Design review of the part built by this model. Coordinates are the model's own, in mm. Face numbers are marked on the shaded views. A direction names the side the tool comes from. Coordinates: 2 decimals unless noted, no trailing zeros.
Q1. The part is to be moulded in two halves that separate along X. For the marked faces 1, 2 and 3, say which applies: released by +X, released by -X, zero draft, split by the parting line, or undercut.
Q2. For pin 1 Ø1 at (x, z) = (12, -10.5) entering from +Y; pin 2 Ø11.5 at (x, y) = (2, 37) entering from -Z; pin 3 Ø0.6 at (x, z) = (1.5, 24.5) entering from +Y; pin 4 Ø3 at (y, z) = (5, 0) entering from +X, all flat-tipped, find the tip position at first contact; note any pin that passes through.
Q3. For the marked faces 4, 5 and 6, list the 3-axis set-ups (+Z, -Z, +X, -X, +Y, -Y) from which the entire face can be reached by the end or side of a thin tool; tool diameter is ignored.
Q4. For L1, parallel to Z at x = 22.45, y = 5 (3 decimals); L2, parallel to X at y = 8, z = 0; L3, parallel to X at y = 26, z = -15, list the stretches that pass through material, from the lowest coordinate up.
from build123d import *

# Parameters (mm, degrees)
SKETCH1_R               = 25
SKETCH1_R_2             = 20.15
BOSS_EXTRUDE1_DEPTH     = 10
SKETCH2_R               = 25
BOSS_EXTRUDE2_DEPTH     = 5
BOSS_EXTRUDE3_DEPTH     = 50
CUT_EXTRUDE1_DEPTH      = 50
SKETCH5_W               = 44
SKETCH5_H               = 33.5
CUT_EXTRUDE2_DEPTH      = 2.33
SKETCH6_W               = 31.902194282
SKETCH6_H               = 10.372222151
BOSS_EXTRUDE5_DEPTH     = 45
BOSS_EXTRUDE6_DEPTH     = 45
BOSS_EXTRUDE7_DEPTH     = 20
SKETCH10_R              = 1.375
CUT_EXTRUDE3_DEPTH      = 77
SKETCH11_R              = 1.375
CUT_EXTRUDE4_DEPTH      = 77
SKETCH12_R              = 3
CUT_EXTRUDE5_DEPTH      = 7.38
CUT_EXTRUDE6_DEPTH      = 7.88
CUT_EXTRUDE6_DEPTH_BACK = 7.38
SKETCH13_R              = 3
CHAMFER1_SIZE           = 30
CHAMFER1_SIZE_2         = 5.289809421
CUT_EXTRUDE7_DEPTH      = 37
CUT_EXTRUDE7_DEPTH_BACK = 37
SKETCH16_R              = 1.625


with BuildPart() as part:
    # Sketch1 → Boss-Extrude1 (new body)
    with BuildSketch(Plane(origin=(0, 0, 0), x_dir=(1, 0, 0), z_dir=(0, 1, 0))):
        with Locations(Location((0, 0, 0), (0, 0, 270))):
            Circle(SKETCH1_R)
        with Locations(Location((0, 0, 0), (0, 0, 270))):
            Circle(SKETCH1_R_2, mode=Mode.SUBTRACT)
    extrude(amount=BOSS_EXTRUDE1_DEPTH)

    # Sketch2 → Boss-Extrude2 (add)
    with BuildSketch(Plane(origin=(0, 10, 0), x_dir=(1, 0, 0), z_dir=(0, 1, 0))):
        with Locations(Location((0, 0, 0), (0, 0, 270))):
            Circle(SKETCH2_R)
    extrude(amount=BOSS_EXTRUDE2_DEPTH)

    # Sketch3 → Boss-Extrude3 (add)
    with BuildSketch(Plane(origin=(0, 15, 0), x_dir=(1, 0, 0), z_dir=(0, 1, 0))):
        with BuildLine():
            ThreePointArc((4.974937186, -24.5), (12.844564237, -21.448010853), (19.25, -15.951097141))
            Line((19.25, -15.951097141), (19.25, 15.951097141))
            ThreePointArc((19.25, 15.951097141), (12.844564237, 21.448010853), (4.974937186, 24.5))
            Line((4.974937186, 24.5), (-4.974937186, 24.5))
            ThreePointArc((-4.974937186, 24.5), (-12.844564237, 21.448010853), (-19.25, 15.951097141))
            Line((-19.25, 15.951097141), (-19.25, -15.951097141))
            ThreePointArc((-19.25, -15.951097141), (-12.844564237, -21.448010853), (-4.974937186, -24.5))
            Line((-4.974937186, -24.5), (4.974937186, -24.5))
        make_face()
    extrude(amount=BOSS_EXTRUDE3_DEPTH)

    # Sketch4 → Cut-Extrude1 (cut)
    with BuildSketch(Plane.XY.offset(24.5)):
        Polygon((-4.974937186, 44.974937186), (4.974937186, 35.025062814), (4.974937186, 65), (-4.974937186, 65), align=None)
        Polygon((4.974937186, 35.025062814), (25, 15), (25, 65), (4.974937186, 65), align=None)
        Polygon((-19.25, 59.25), (-4.974937186, 44.974937186), (-4.974937186, 65), (-19.25, 65), align=None)
    extrude(amount=-CUT_EXTRUDE1_DEPTH, mode=Mode.SUBTRACT)

    # Sketch5 → Cut-Extrude2 (cut)
    # profile 1 of 2: a face of its own
    with BuildSketch(Plane(origin=(20, 20, 0), x_dir=(0, 0, -1), z_dir=(0.7071067811865485, 0.7071067811865467, 0))):
        with BuildLine():
            Line((21.978674947, 45.132882323), (-21.978674947, 45.132882323))
            add(Edge.make_bspline(
                [(-21.978674947, 45.132882323), (-22.0399199, 44.9730967), (-22.1, 44.81242904)],
                knots=[4.215256564, 4.215256564, 4.215256564, 4.225444941, 4.225444941, 4.225444941], degree=2, weights=[0.971948047, 0.972055152, 0.97218796]))
            Line((-22.1, 44.81242904), (-22.1, 11.756113455))
            add(Edge.make_bspline(
                [(-22.1, 11.756113455), (-22.039397631, 11.594049133), (-21.977610099, 11.432882323)],
                knots=[5.19933302, 5.19933302, 5.19933302, 5.20960995, 5.20960995, 5.20960995], degree=2, weights=[0.97218796, 0.972053998, 0.971946187]))
            Line((-21.977610099, 11.432882323), (21.977610099, 11.432882323))
            add(Edge.make_bspline(
                [(21.977610099, 11.432882323), (22.039397631, 11.594049133), (22.1, 11.756113455)],
                knots=[1.073575357, 1.073575357, 1.073575357, 1.083852287, 1.083852287, 1.083852287], degree=2, weights=[0.971946187, 0.972053998, 0.97218796]))
            Line((22.1, 11.756113455), (22.1, 44.81242904))
            add(Edge.make_bspline(
                [(22.1, 44.81242904), (22.0399199, 44.9730967), (21.978674947, 45.132882323)],
                knots=[2.057740366, 2.057740366, 2.057740366, 2.067928743, 2.067928743, 2.067928743], degree=2, weights=[0.97218796, 0.972055152, 0.971948047]))
        make_face()
        with Locations((0, 28.282882323)):
            Rectangle(SKETCH5_W, SKETCH5_H, mode=Mode.SUBTRACT)
    # profile 2 of 2: a face of its own
    with BuildSketch(Plane(origin=(20, 20, 0), x_dir=(0, 0, -1), z_dir=(0.7071067811865485, 0.7071067811865467, 0))):
        with Locations((0, 28.282882323)):
            Rectangle(SKETCH5_W, SKETCH5_H)
    extrude(amount=-CUT_EXTRUDE2_DEPTH, mode=Mode.SUBTRACT)

    # Sketch6 → Boss-Extrude5 (add)
    with BuildSketch(Plane(origin=(20, 20, 0), x_dir=(0, 0, -1), z_dir=(0.7071067811865487, 0.7071067811865465, 0))):
        with BuildLine():
            Line((-15.951097141, 1.060660172), (-15.951097141, 11.432882323))
            Line((-15.951097141, 11.432882323), (-21.977610099, 11.432882323))
            add(Edge.make_bspline(
                [(-21.977610099, 11.432882323), (-19.67346685, 5.422747233), (-15.951097141, 1.060660172)],
                knots=[5.209205396, 5.209205396, 5.209205396, 5.591230132, 5.591230132, 5.591230132], degree=2, weights=[1, 0.981812537, 1]))
        make_face()
        with Locations((0, 6.246771248)):
            Rectangle(SKETCH6_W, SKETCH6_H)
        with BuildLine():
            Line((21.977610099, 11.432882323), (15.951097141, 11.432882323))
            Line((15.951097141, 11.432882323), (15.951097141, 1.060660172))
            add(Edge.make_bspline(
                [(15.951097141, 1.060660172), (19.67346685, 5.422747233), (21.977610099, 11.432882323)],
                knots=[0.691955175, 0.691955175, 0.691955175, 1.073979912, 1.073979912, 1.073979912], degree=2, weights=[1, 0.981812537, 1]))
        make_face()
    extrude(amount=BOSS_EXTRUDE5_DEPTH)

    # Sketch7 → Boss-Extrude6 (add)
    with BuildSketch(Plane(origin=(20, 20, 0), x_dir=(0, 0, -1), z_dir=(0.7071067811865487, 0.7071067811865465, 0))):
        with BuildLine():
            Line((15.951097141, 55.507882323), (-15.951097141, 55.507882323))
            add(Edge.make_bspline(
                [(-15.951097141, 55.507882323), (-19.67435923, 51.144749519), (-21.978674947, 45.132882323)],
                knots=[3.833547829, 3.833547829, 3.833547829, 4.215661937, 4.215661937, 4.215661937], degree=2, weights=[1, 0.981804052, 1]))
            Line((-21.978674947, 45.132882323), (21.978674947, 45.132882323))
            add(Edge.make_bspline(
                [(21.978674947, 45.132882323), (19.67435923, 51.144749519), (15.951097141, 55.507882323)],
                knots=[2.06752337, 2.06752337, 2.06752337, 2.449637478, 2.449637478, 2.449637478], degree=2, weights=[1, 0.981804052, 1]))
        make_face()
    extrude(amount=BOSS_EXTRUDE6_DEPTH)

    # Sketch8 → Boss-Extrude7 (add)
    with BuildSketch(Plane(origin=(0, 15, 0), x_dir=(1, 0, 0), z_dir=(0, 1, 0))):
        with BuildLine():
            ThreePointArc((25, 0), (23.518609653, 8.477912479), (19.25, 15.951097141))
            Line((19.25, 15.951097141), (19.25, -15.951097141))
            ThreePointArc((19.25, -15.951097141), (23.518609653, -8.477912479), (25, 0))
        make_face()
    extrude(amount=BOSS_EXTRUDE7_DEPTH)

    # Sketch10 → Cut-Extrude3 (cut)
    with BuildSketch(Plane(origin=(-39.25, 39.25, 0), x_dir=(0, 0, 1), z_dir=(-0.7071067811865464, 0.7071067811865487, 0))):
        with Locations(Location((8.001097141, 32.704271247, 0), (0, 0, 270))):
            Circle(SKETCH10_R)
        with Locations(Location((-7.998902859, 32.704271247, 0), (0, 0, 270))):
            Circle(SKETCH10_R)
    extrude(amount=-CUT_EXTRUDE3_DEPTH, mode=Mode.SUBTRACT)

    # Sketch11 → Cut-Extrude4 (cut)
    with BuildSketch(Plane(origin=(-39.25, 39.25, 0), x_dir=(0, 0, 1), z_dir=(-0.7071067811865464, 0.7071067811865487, 0))):
        with Locations(Location((-7.998902859, 64.704271247, 0), (0, 0, 270))):
            Circle(SKETCH11_R)
        with Locations(Location((8.001097141, 64.704271247, 0), (0, 0, 270))):
            Circle(SKETCH11_R)
    extrude(amount=-CUT_EXTRUDE4_DEPTH, mode=Mode.SUBTRACT)

    # Sketch12 → Cut-Extrude5 (cut)
    with BuildSketch(Plane(origin=(-39.25, 39.25, 0), x_dir=(0, 0, 1), z_dir=(-0.7071067811865464, 0.7071067811865487, 0))):
        with Locations(Location((-7.998902859, 64.704271247, 0), (0, 0, 270))):
            Circle(SKETCH12_R)
        with Locations(Location((8.001097141, 64.704271247, 0), (0, 0, 270))):
            Circle(SKETCH12_R)
        with Locations(Location((-7.998902859, 32.704271247, 0), (0, 0, 270))):
            Circle(SKETCH12_R)
        with Locations(Location((8.001097141, 32.704271247, 0), (0, 0, 270))):
            Circle(SKETCH12_R)
    extrude(amount=-CUT_EXTRUDE5_DEPTH, mode=Mode.SUBTRACT)

    # Sketch13 → Cut-Extrude6 (cut, two sides: drawn at the far end of the back side and taken through both)
    with BuildSketch(Plane(origin=(-0.75, 0.75, 0), x_dir=(0, 0, -1), z_dir=(0.7071067811865464, -0.7071067811865487, 0)).offset(-CUT_EXTRUDE6_DEPTH_BACK)):
        with Locations(Location((-8.001097141, 64.704271247, 0), (0, 0, 270))):
            Circle(SKETCH13_R)
        with Locations(Location((7.998902859, 64.704271247, 0), (0, 0, 270))):
            Circle(SKETCH13_R)
        with Locations(Location((-8.001097141, 32.704271247, 0), (0, 0, 270))):
            Circle(SKETCH13_R)
        with Locations(Location((7.998902859, 32.704271247, 0), (0, 0, 270))):
            Circle(SKETCH13_R)
    extrude(amount=CUT_EXTRUDE6_DEPTH + CUT_EXTRUDE6_DEPTH_BACK, mode=Mode.SUBTRACT)

    # Chamfer1
    # the kernel refuses this chamfer: 30, 5.289809421 mm, written as the material it takes off along each edge
    with BuildSketch(Plane(origin=(51.069805153, 52.569805153, 93.907261034), x_dir=(-0.7023657291994666, -0.7118162560985113, 0), z_dir=(0, 0, -1)), Plane(origin=(12.569805153, 91.069805153, -93.907261034), x_dir=(-0.7118162560985133, -0.7023657291994647, 0), z_dir=(0, 0, 1))) as chamfer1_piece_1:
        Polygon((CHAMFER1_SIZE * 0.999977671636, CHAMFER1_SIZE * 0.0066825316561), (-CHAMFER1_SIZE_2 * 0.00668253165642, CHAMFER1_SIZE_2 * 0.999977671684), (0, 0), align=None)
    extrude(amount=187.814522067, mode=Mode.SUBTRACT)

    # Sketch16 → Cut-Extrude7 (cut, two sides: drawn at the far end of the back side and taken through both)
    with BuildSketch(Plane(origin=(0, 0, 0), x_dir=(0, 0, -1), z_dir=(1, 0, 0)).offset(-CUT_EXTRUDE7_DEPTH_BACK)):
        with Locations(Location((0, 5, 0), (0, 0, 180))):
            Circle(SKETCH16_R)
    extrude(amount=CUT_EXTRUDE7_DEPTH + CUT_EXTRUDE7_DEPTH_BACK, mode=Mode.SUBTRACT)


solid = part.part
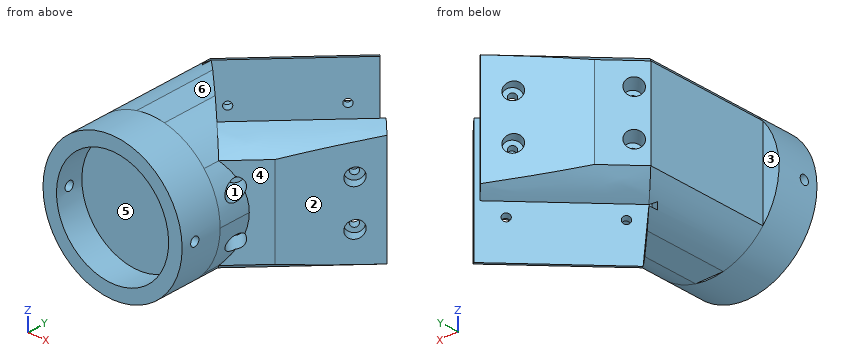
Responses:
1. face 1: undercut
1. face 2: released by +X
1. face 3: zero draft
2. pin 1: stops at y = 84.66
2. pin 2: stops at z = -24.5
2. pin 3: stops at y = 38.8
2. pin 4: passes through
3. face 4: +X, -Y
3. face 5: -Y
3. face 6: +Z, +X, -X, +Y
4. L1: z = -11 to -1.625, 1.625 to 11
4. L2: x = -25 to -20.15, 20.15 to 25
4. L3: x = -19.25 to 24.5
